from build123d import *

# Parameters (mm, degrees)
SKETCH1_W               = 39.624
SKETCH1_H               = 63.5
BOSS_EXTRUDE1_DEPTH     = 1.5875
SKETCH2_W               = 39.624
SKETCH2_H               = 3.175
BOSS_EXTRUDE2_DEPTH     = 6.35
SKETCH3_R               = 6.35
CUT_EXTRUDE1_DEPTH      = 8.9375
CUT_EXTRUDE2_DEPTH      = 1
CUT_EXTRUDE2_DEPTH_BACK = 8.9375
SKETCH5_W               = 12.7
SKETCH5_H               = 28.946652836
CUT_EXTRUDE3_DEPTH      = 8.9375
SKETCH6_W               = 13.462
SKETCH6_H               = 12.7
BOSS_EXTRUDE3_DEPTH     = 1.5875
SKETCH7_W               = 7.112
SKETCH7_H               = 6.35
CUT_EXTRUDE4_DEPTH      = 77.2
FILLET1_R               = 3.175
F_4_CLEARANCE_HOLE1_D   = 2.9464
SKETCH10_R              = 2.38125
CUT_EXTRUDE5_DEPTH      = 74.025


with BuildPart() as part:
    # Sketch1 → Boss-Extrude1 (new body)
    with BuildSketch(Plane(origin=(0, 0, 0), x_dir=(1, 0, 0), z_dir=(0, 1, 0))):
        with Locations((0, -31.75)):
            Rectangle(SKETCH1_W, SKETCH1_H)
    extrude(amount=BOSS_EXTRUDE1_DEPTH)

    # Sketch2 → Boss-Extrude2 (add)
    with BuildSketch(Plane.XZ):
        with Locations((0, 1.5875)):
            Rectangle(SKETCH2_W, SKETCH2_H)
    extrude(amount=BOSS_EXTRUDE2_DEPTH)

    # Sketch3 → Cut-Extrude1 (cut, through all)
    with BuildSketch(Plane(origin=(10.289309191, 1.5875, 36.06936054), x_dir=(1, 0, 0), z_dir=(0, 1, 0))):
        with Locations((-10.289309191, -3.379645711)):
            Circle(SKETCH3_R)
    extrude(amount=-CUT_EXTRUDE1_DEPTH, mode=Mode.SUBTRACT)

    # Sketch4 → Cut-Extrude2 (cut, two sides)
    with BuildSketch(Plane(origin=(0, 1.5875, 0), x_dir=(1, 0, 0), z_dir=(0, 1, 0))) as cut_extrude2_sk:
        Polygon((-19.812, -38.1), (5.588, -63.5), (-19.812, -63.5), align=None)
    extrude(amount=CUT_EXTRUDE2_DEPTH, mode=Mode.SUBTRACT)
    extrude(cut_extrude2_sk.sketch, amount=-CUT_EXTRUDE2_DEPTH_BACK, mode=Mode.SUBTRACT)

    # Sketch5 → Cut-Extrude3 (cut, through all)
    with BuildSketch(Plane(origin=(0, 1.5875, 0), x_dir=(1, 0, 0), z_dir=(0, 1, 0))):
        with Locations((0, -53.922332669)):
            Rectangle(SKETCH5_W, SKETCH5_H)
    extrude(amount=-CUT_EXTRUDE3_DEPTH, mode=Mode.SUBTRACT)

    # Sketch6 → Boss-Extrude3 (add)
    with BuildSketch(Plane(origin=(0, 1.5875, 0), x_dir=(1, 0, 0), z_dir=(0, 1, 0))):
        with Locations((13.081, -69.85)):
            Rectangle(SKETCH6_W, SKETCH6_H)
    extrude(amount=-BOSS_EXTRUDE3_DEPTH)

    # Sketch7 → Cut-Extrude4 (cut, through all)
    with BuildSketch(Plane(origin=(0, 0, 0), x_dir=(-1, 0, 0), z_dir=(0, 0, -1))):
        with Locations((-16.256, -3.175)):
            Rectangle(SKETCH7_W, SKETCH7_H)
        with Locations((16.256, -3.175)):
            Rectangle(SKETCH7_W, SKETCH7_H)
    extrude(amount=-CUT_EXTRUDE4_DEPTH, mode=Mode.SUBTRACT)

    # Fillet1
    fillet1_edges = [part.edges().sort_by_distance(p)[0] for p in [
        (-12.7, 0, 1.5875),
        (0, 0, 3.175),
        (12.7, 0, 1.5875),
    ]]
    fillet(fillet1_edges, radius=FILLET1_R)

    # #4 Clearance Hole1 (through all)
    with Locations(Plane(origin=(0, 0, 0), x_dir=(-1, 0, 0), z_dir=(0, 0, -1))):
        with Locations((-9.525, -3.175), (9.525, -3.175)):
            Hole(F_4_CLEARANCE_HOLE1_D / 2)

    # Sketch10 → Cut-Extrude5 (cut, through all)
    with BuildSketch(Plane.XY.offset(3.175)):
        with Locations((9.525, -3.175)):
            Circle(SKETCH10_R)
        with Locations((-9.525, -3.175)):
            Circle(SKETCH10_R)
    extrude(amount=CUT_EXTRUDE5_DEPTH, mode=Mode.SUBTRACT)


solid = part.part
Could you check a few things on this model? Use its own coordinates, in mm. A direction names the side the tool comes from. Give positions to 0.01 mm unless a question says otherwise; leave off trailing zeros. Order: outer loops, then holes, each group sorted by start corner. A loop starts at its lowest first (then second) coordinate and runs counter-clockwise, first axis right, second up.
1. Suppose I cut it at D-D (z = 56). List the corners of the cut face in (x, y) for me.
2. I need wall thicknesses on L1, parallel to X at y = 1, z = 66; L2, parallel to Z at x = -2, y = -5.25 (3 decimals); L3, parallel to Y at x = 17, z = 45. Which ranges of each line are inside material? Lowest first, please.
3. Suppose I cut it at B-B (z = 36). List the corners of the cut face in (x, y) for me, plus the area to 3 significant figures.
4. We'd pull the mould along X, two halves only. Please class faces 1 (the cylindrical face through (-10.997, -3.11, 1.61)), 2 (the cylindrical face through (14.03, -0.59, 2.51)), 3 (the flat face through (-6.35, 1, 46)), 4 (the flat face through (13, 1, 76.2)): pulls with the +X half, pulls with the -X half, needs draft (parallel to the pull), parting line crosses it, or undercut.
5. Will these pins go through, and if not, where does the flat tip stop? P1, Ø3.5, axis at x = 9.525, y = -3.175, coming from the -Z side; P2, Ø1.6, axis at y = -5.5, z = 2, coming from the +X side; P3, Ø1.3, axis at y = 0.5, z = 53.5, coming from the -X side; P4, Ø6, axis at x = 11.5, z = 60, coming from the -Y side.
6. For faces 5 (the cylindrical face through (9.577, -0.794, 3.586)), 6 (the flat face through (0, -1, 0)), 7 (the flat face through (-12.7, -5, 2)), 8 (the flat face through (6.35, 1, 58)), 9 (the flat face through (12.7, -5, 2)), which set-ups out of +Z, -Z, +X, -X, +Y, -Y let a thin tool reach every point of the face, with its end or its side?
Solved:
1. outline: (6.35, 0) - (19.81, 0) - (19.81, 1.59) - (6.35, 1.59) - close
2. L1: x = 6.35 to 19.81
2. L2: z = 0 to 3.175
2. L3: y = 0 to 1.59
3. outline: (-19.81, 0) - (-5.33, 0) - (-5.33, 1.59) - (-19.81, 1.59) - close; (5.33, 0) - (19.81, 0) - (19.81, 1.59) - (5.33, 1.59) - close
3. area: 46.0 mm2
4. face 1: undercut
4. face 2: pulls with the +X half
4. face 3: undercut
4. face 4: needs draft
5. P1: stops at z = 0
5. P2: stops at x = 12.7
5. P3: stops at x = 6.35
5. P4: stops at y = 0
6. face 5: +Z, -Y
6. face 6: -Z, +X, -X, +Y, -Y
6. face 7: +Z, -Z, -X, -Y
6. face 8: +Z, +Y, -Y
6. face 9: +Z, -Z, +X, -Y
